Input: part model. Units: mm. Frame: model coordinates. A direction names the side the tool comes from. Give positions to 0.01 mm unless a question says otherwise; leave off trailing zeros. Loops run counter-clockwise (first coordinate to the right, second up) from the corner with the lowest first, then second, coordinate; pieces in that order, holes last.
from build123d import *

# Parameters (mm, degrees)
SKETCH1_W           = 15
SKETCH1_H           = 10.5
SKETCH1_W_2         = 15.8
SKETCH1_H_2         = 2
BOSS_EXTRUDE1_DEPTH = 2.3
SKETCH1_2_W         = 15.8
SKETCH1_2_H         = 2
BOSS_EXTRUDE2_DEPTH = 1.25


with BuildPart() as part:
    # Sketch1 → Boss-Extrude1 (new body)
    with BuildSketch(Plane.XY):
        Polygon((0, 0), (0, -2), (2.5, -2), (2.5, 0), (17.5, 0), (17.5, -2), (20, -2), (20, 0), (20, 18), (0, 18), align=None)
        with Locations((10, 7.75)):
            Rectangle(SKETCH1_W, SKETCH1_H, mode=Mode.SUBTRACT)
        with Locations((10, 15.5)):
            Rectangle(SKETCH1_W_2, SKETCH1_H_2, mode=Mode.SUBTRACT)
    extrude(amount=BOSS_EXTRUDE1_DEPTH)

    # Sketch1<2> → Boss-Extrude2 (add)
    with BuildSketch(Plane.XY):
        with Locations((10, 15.5)):
            Rectangle(SKETCH1_2_W, SKETCH1_2_H)
    extrude(amount=BOSS_EXTRUDE2_DEPTH)


solid = part.part
(1) Cut plane A-A (z = 1.85). Return the cut outline in (x, y), and give its area (3 significant figures).
Values follow:
outline: (0, -2) - (2.5, -2) - (2.5, 0) - (17.5, 0) - (17.5, -2) - (20, -2) - (20, 18) - (0, 18) - close; hole (2.1, 14.5) - (17.9, 14.5) - (17.9, 16.5) - (2.1, 16.5) - close; hole (2.5, 2.5) - (17.5, 2.5) - (17.5, 13) - (2.5, 13) - close
area: 181 mm2
(2) Reachability of faces 1 (the flat face through (10, 18, 1)), 2 (the flat face through (10, 14.5, 2)), 3 (the flat face through (2.5, -1, 1)), 4 (the flat face through (17.5, 8, 1)) from +Z, -Z, +X, -X, +Y, -Y: full face, straight path, thin tool, end or side. Return the list, or none.
Values follow:
face 1: +Z, -Z, +X, -X, +Y
face 2: +Z
face 3: +Z, -Z, -Y
face 4: +Z, -Z
(3) Ray query, probe 1 along Y at (x, z) = (11, 2); probe 2 along X at (y, z) = (5, 1.3); probe 3 along Y at (x, z) = (6, 0.75). Return the intervals inside material, ascending.
Values follow:
probe 1: y = 0 to 2.5, 13 to 14.5, 16.5 to 18
probe 2: x = 0 to 2.5, 17.5 to 20
probe 3: y = 0 to 2.5, 13 to 18
(4) Cut plane D-D (y = 8.25). Return the cut outline in (x, z), and give its area (3 significant figures).
Values follow:
outline: (0, 0) - (2.5, 0) - (2.5, 2.3) - (0, 2.3) - close; (17.5, 0) - (20, 0) - (20, 2.3) - (17.5, 2.3) - close
area: 11.5 mm2
(5) Pin query (flat end, axial travel): pin 1 Ø0.7 at (x, z) = (13.5, 0.5) entering from -Y; pin 2 Ø1.6 at (x, y) = (7.5, 15.5) entering from +Z; pin 3 Ø1 at (y, z) = (8.5, 2) entering from -X; pin 4 Ø1.5 at (x, y) = (7.5, 11.5) entering from +Z. Return the tip coordinate at first contact, or that it passes through.
Values follow:
pin 1: stops at y = 0
pin 2: stops at z = 1.25
pin 3: stops at x = 0
pin 4: passes through
(6) Cut plane C-C (x = 13). Return the cut outline in (y, z).
Values follow:
outline: (0, 0) - (2.5, 0) - (2.5, 2.3) - (0, 2.3) - close; (13, 0) - (18, 0) - (18, 2.3) - (16.5, 2.3) - (16.5, 1.25) - (14.5, 1.25) - (14.5, 2.3) - (13, 2.3) - close
(7) Mould query, pull axis Y, two halves, no side actions, for faces 5 (the flat face through (10, 1, 2.3)), 6 (the flat face through (10, 2.5, 1)), 7 (the flat face through (10, 0, 1)). Classes: +Y half, -Y half, draft (parallel to the pull), parting line (faces both ways), or undercut.
Values follow:
face 5: draft
face 6: undercut
face 7: -Y half
(8) Cut plane B-B (z = 0.4). Return the cut outline in (x, y), and give its area (4 significant figures).
Values follow:
outline: (0, -2) - (2.5, -2) - (2.5, 0) - (17.5, 0) - (17.5, -2) - (20, -2) - (20, 18) - (0, 18) - close; hole (2.5, 2.5) - (17.5, 2.5) - (17.5, 13) - (2.5, 13) - close
area: 212.5 mm2
